```python
from build123d import *

# Parameters (mm, degrees)
F0_W     = 101.6
F0_H     = 38.1
F1_DEPTH = 12.7
F3_D     = 3.175
F3_DEPTH = 9.525
F3_TIP   = 0.9538662327


with BuildPart() as f1:
    # F0 (on Top) → F1 (new body)
    with BuildSketch(Plane.XY):
        Rectangle(F0_W, F0_H)
    extrude(amount=F1_DEPTH)

    # F3
    with Locations(Plane.XY.offset(12.7)):
        with Locations((9.525, 9.525), (34.925, 9.525), (34.925, -9.525), (9.525, -9.525)):
            Hole(F3_D / 2, depth=F3_DEPTH)
            with Locations((0, 0, -(F3_DEPTH + F3_TIP / 2))):  # 118° drill point
                Cone(0, F3_D / 2, F3_TIP, mode=Mode.SUBTRACT)


solid = f1.part
```
Geometry: final body of the model. Coordinates: model frame, mm. A direction names the side the tool comes from. Coordinates: 2 decimals unless noted, no trailing zeros. Write each question's results on one line, items separated by ' | '.
1) Pin query (flat end, axial travel): pin 1 (1.9 mm diameter, centred on x = 9.525, y = -9.525, fed in from +Z); pin 2 (2.5 mm diameter, centred on x = 34.925, y = -9.525, fed in from +Z); pin 3 (3 mm diameter, centred on x = 9.525, y = 9.525, fed in from +Z). Return the tip coordinate at first contact, or that it passes through.
Results list:
pin 1: z = 2.79 | pin 2: z = 2.97 | pin 3: z = 3.12
2) Set-up query: faces 5 (the cylindrical face through (36.51, -9.46, 7.87)), 6 (the flat face through (-1, 0, 0)). Return all of +Z, -Z, +X, -X, +Y, -Y with unobstructed straight access to the full face (end or side cutting, diameter ignored); none if empty.
Results list:
face 5: +Z | face 6: -Z, +X, -X, +Y, -Y
3) Line query: line 1 (X direction, y = 10, z = 4.75); line 2 (X direction, y = -8.5, z = 5.75). Output: solid intervals per line, ascending. Write a range as from..to.
Results list:
line 1: -50.8..8.01, 11.04..33.41, 36.44..50.8 | line 2: -50.8..8.31, 10.74..33.71, 36.14..50.8
4) Pull-direction query (X, two-part tool) for faces 1 (the conical face through (34.65, 9.537, 2.387)), 2 (the flat face through (-1, 0, 12.7)), 3 (the flat face through (-50.8, 0, 6)), 4 (the conical face through (9.306, 9.357, 2.387)); classes: pulls with the +X half, pulls with the -X half, needs draft (parallel to the pull), parting line crosses it, or undercut.
Results list:
face 1: undercut | face 2: needs draft | face 3: pulls with the -X half | face 4: undercut
